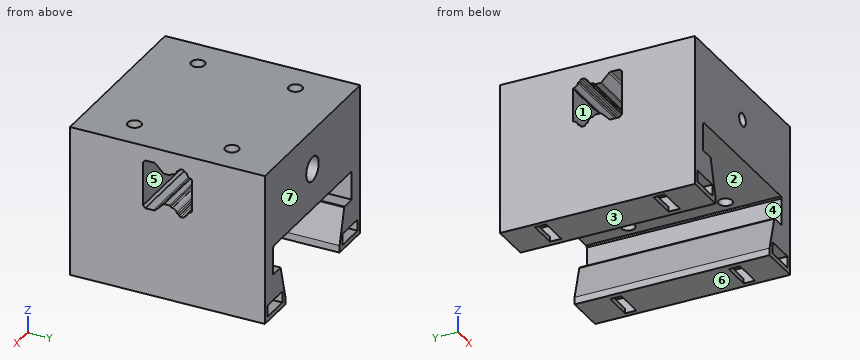
from build123d import *

# Parameters (mm, degrees)
SKETCH1_W           = 57
SKETCH1_H           = 28.7
BOSS_EXTRUDE1_DEPTH = 60
SKETCH2_W           = 9
SKETCH2_H           = 4
CUT_EXTRUDE1_DEPTH  = 69.064473112
BOSS_EXTRUDE2_DEPTH = 28.5
SKETCH6_W           = 15.5
SKETCH6_H           = 15.390476131
CUT_EXTRUDE2_DEPTH  = 80
BOSS_EXTRUDE5_DEPTH = 60
SKETCH10_R          = 2.1
CUT_EXTRUDE3_DEPTH  = 24.530533394
SKETCH11_W          = 61.984050455
SKETCH11_H          = 43.227353824
SKETCH11_W_2        = 6
SKETCH11_H_2        = 2.542732203
CUT_EXTRUDE4_DEPTH  = 77.839254789
SKETCH13_W          = 6.011053281
SKETCH13_H          = 2.620549071
CUT_EXTRUDE5_DEPTH  = 77.839254789
SKETCH14_W          = 9
SKETCH14_H          = 4
BOSS_EXTRUDE7_DEPTH = 60
SKETCH12_W          = 10.230058637
SKETCH12_H          = 6.686923691
BOSS_EXTRUDE6_DEPTH = 60
SKETCH15_W          = 9
SKETCH15_H          = 4
BOSS_EXTRUDE8_DEPTH = 60
SKETCH16_W          = 9
SKETCH16_H          = 1.78
CUT_EXTRUDE6_DEPTH  = 77.839254789
SKETCH17_W          = 25.75
SKETCH17_H          = 20.1006285
CUT_EXTRUDE7_DEPTH  = 77.839254789
SKETCH18_W          = 32.4
SKETCH18_H          = 12.613288226
CUT_EXTRUDE8_DEPTH  = 75.79485996
SKETCH19_W          = 57
SKETCH19_H          = 3.949842852
CUT_EXTRUDE9_DEPTH  = 75.79485996
SKETCH20_W          = 9
SKETCH20_H          = 3.5
CUT_EXTRUDE10_DEPTH = 75.79485996
SKETCH21_W          = 9
SKETCH21_H          = 3.5
CUT_EXTRUDE11_DEPTH = 1.5
SKETCH23_R          = 3.75
CUT_EXTRUDE12_DEPTH = 59.313986952
SKETCH24_R          = 2
CUT_EXTRUDE13_DEPTH = 59.313986952


with BuildPart() as part:
    # Sketch1 → Boss-Extrude1 (new body)
    with BuildSketch(Plane(origin=(0, 0, 0), x_dir=(1, 0, 0), z_dir=(0, 1, 0))):
        with Locations((0, -0.5)):
            Rectangle(SKETCH1_W, SKETCH1_H)
        Polygon((23.07, -9.85), (-23.07, -9.85), (-23.5, -9.42), (-23.5, -0.95), (-19.09385128, -0.95), (-19, -0.599742255), (-16.2, 9.85), (16.2, 9.85), (19, -0.599742255), (19.09385128, -0.95), (23.5, -0.95), (23.5, -2.9), (23.5, -9.42), align=None, mode=Mode.SUBTRACT)
    extrude(amount=BOSS_EXTRUDE1_DEPTH)

    # Sketch2 → Cut-Extrude1 (cut, through all)
    with BuildSketch(Plane.XZ):
        with Locations((24, -10.0706285)):
            Rectangle(SKETCH2_W, SKETCH2_H)
        with Locations((-24, -10.0706285)):
            Rectangle(SKETCH2_W, SKETCH2_H)
    extrude(amount=-CUT_EXTRUDE1_DEPTH, mode=Mode.SUBTRACT)

    # Sketch5 → Boss-Extrude2 (add, symmetric)
    with BuildSketch(Plane(origin=(0, 0, 0), x_dir=(0, 0, -1), z_dir=(1, 0, 0))):
        with BuildLine():
            Line((-14.85, 0), (-14.85, 23.200000017))
            Line((-14.85, 23.200000017), (-15.549999973, 22.50000003))
            Line((-15.549999973, 22.50000003), (-29.149999973, 22.50000003))
            Line((-29.149999973, 22.50000003), (-29.849999973, 23.20000003))
            Line((-29.849999973, 23.20000003), (-29.849999973, 25.743360053))
            ThreePointArc((-29.849999973, 25.743360053), (-29.773879502, 26.126043492), (-29.557106746, 26.450466847))
            Line((-29.557106746, 26.450466847), (-27.237157266, 28.770416328))
            ThreePointArc((-27.237157266, 28.770416328), (-27.150448162, 28.900185674), (-27.119999973, 29.053259055))
            Line((-27.119999973, 29.053259055), (-27.119999973, 30.615319642))
            ThreePointArc((-27.119999973, 30.615319642), (-27.150448164, 30.768393021), (-27.237157268, 30.898162365))
            Line((-27.237157268, 30.898162365), (-27.431588163, 31.09259326))
            ThreePointArc((-27.431588163, 31.09259326), (-27.613507965, 31.297692563), (-27.620638933, 31.57175403))
            ThreePointArc((-27.620638933, 31.57175403), (-28.017573243, 32.42857618), (-28.828543655, 32.91234062))
            ThreePointArc((-28.828543655, 32.91234062), (-29.01918836, 33.020436377), (-29.124259054, 33.212764861))
            Line((-29.124259054, 33.212764861), (-29.156235284, 33.354092333))
            ThreePointArc((-29.156235284, 33.354092333), (-29.24659278, 33.53064407), (-29.410649592, 33.642090719))
            Line((-29.410649592, 33.642090719), (-29.585724304, 33.70524196))
            ThreePointArc((-29.585724304, 33.70524196), (-29.777329878, 33.851609246), (-29.849999973, 34.081511694))
            Line((-29.849999973, 34.081511694), (-29.849999973, 34.837490602))
            ThreePointArc((-29.849999973, 34.837490602), (-29.772088513, 35.074680338), (-29.568705112, 35.219471078))
            Line((-29.568705112, 35.219471078), (-29.427668799, 35.263299846))
            ThreePointArc((-29.427668799, 35.263299846), (-29.25116358, 35.375371369), (-29.155313737, 35.561185593))
            Line((-29.155313737, 35.561185593), (-29.125010632, 35.702102112))
            ThreePointArc((-29.125010632, 35.702102112), (-29.020526118, 35.897067182), (-28.828406063, 36.006695082))
            ThreePointArc((-28.828406063, 36.006695082), (-28.025619489, 36.481556021), (-27.62403672, 37.32339358))
            ThreePointArc((-27.62403672, 37.32339358), (-27.540484938, 37.407225271), (-27.43605838, 37.46293655))
            Line((-27.43605838, 37.46293655), (-27.39899493, 37.5))
            Line((-27.39899493, 37.5), (-17.30100503, 37.5))
            Line((-17.30100503, 37.5), (-17.26394158, 37.46293655))
            ThreePointArc((-17.26394158, 37.46293655), (-17.159515017, 37.407225278), (-17.07596324, 37.32339358))
            ThreePointArc((-17.07596324, 37.32339358), (-16.674380468, 36.481556018), (-15.871593887, 36.006695079))
            ThreePointArc((-15.871593887, 36.006695079), (-15.679473839, 35.897067189), (-15.574989331, 35.702102127))
            Line((-15.574989331, 35.702102127), (-15.544686222, 35.561185587))
            ThreePointArc((-15.544686222, 35.561185587), (-15.448836377, 35.375371364), (-15.272331158, 35.263299843))
            Line((-15.272331158, 35.263299843), (-15.131294869, 35.219471083))
            ThreePointArc((-15.131294869, 35.219471083), (-14.927911462, 35.074680333), (-14.85, 34.837490586))
            Line((-14.85, 34.837490586), (-14.85, 60))
            Line((-14.85, 60), (-34.380533394, 60))
            Line((-34.380533394, 60), (-34.380533394, 0))
            Line((-34.380533394, 0), (-14.85, 0))
        make_face()
        with BuildLine():
            ThreePointArc((-15.142893227, 26.450466847), (-14.926120471, 26.126043492), (-14.85, 25.743360053))
            Line((-14.85, 25.743360053), (-14.85, 34.081511674))
            ThreePointArc((-14.85, 34.081511674), (-14.922670087, 33.851609245), (-15.114275644, 33.70524197))
            Line((-15.114275644, 33.70524197), (-15.289350386, 33.642090718))
            ThreePointArc((-15.289350386, 33.642090718), (-15.453407192, 33.53064407), (-15.543764688, 33.354092339))
            Line((-15.543764688, 33.354092339), (-15.57574092, 33.21276486))
            ThreePointArc((-15.57574092, 33.21276486), (-15.680811613, 33.020436377), (-15.871456319, 32.91234062))
            ThreePointArc((-15.871456319, 32.91234062), (-16.68242673, 32.42857618), (-17.07936104, 31.57175403))
            ThreePointArc((-17.07936104, 31.57175403), (-17.086492012, 31.297692565), (-17.26841181, 31.09259326))
            Line((-17.26841181, 31.09259326), (-17.462842708, 30.898162362))
            ThreePointArc((-17.462842708, 30.898162362), (-17.549551812, 30.768393016), (-17.58, 30.615319635))
            Line((-17.58, 30.615319635), (-17.58, 29.053259048))
            ThreePointArc((-17.58, 29.053259048), (-17.54955181, 28.900185669), (-17.462842705, 28.770416325))
            Line((-17.462842705, 28.770416325), (-15.142893227, 26.450466847))
        make_face()
    extrude(amount=BOSS_EXTRUDE2_DEPTH, both=True)

    # Sketch6 → Cut-Extrude2 (cut)
    with BuildSketch(Plane(origin=(0, 60, 0), x_dir=(1, 0, 0), z_dir=(0, 1, 0))):
        with Locations((0, 12.050145064)):
            Rectangle(SKETCH6_W, SKETCH6_H)
    extrude(amount=-CUT_EXTRUDE2_DEPTH, mode=Mode.SUBTRACT)

    # Sketch9 → Boss-Extrude5 (add)
    with BuildSketch(Plane(origin=(0, 60, 0), x_dir=(1, 0, 0), z_dir=(0, 1, 0))):
        Polygon((-19.5, 13.85), (-19.5, 29.1706285), (-28.5, 29.1706285), (-28.5, 26.1706285), (-33.5, 26.1706285), (-33.5, 32.1706285), (-14.5, 32.1706285), (-14.5, 13.85), align=None)
        Polygon((30.2, 12.85), (30.2, 28.735786438), (19.5, 28.735786438), (19.5, 13.85), (14.5, 13.85), (14.5, 32.1706285), (33.5, 32.1706285), (33.5, 12.85), align=None)
    extrude(amount=-BOSS_EXTRUDE5_DEPTH)

    # Sketch10 → Cut-Extrude3 (cut)
    with BuildSketch(Plane.XY.offset(34.380533394)):
        with Locations((19, 45)):
            Circle(SKETCH10_R)
        with Locations((19, 15)):
            Circle(SKETCH10_R)
        with Locations((-19, 15)):
            Circle(SKETCH10_R)
        with Locations((-19, 45)):
            Circle(SKETCH10_R)
    extrude(amount=-CUT_EXTRUDE3_DEPTH, mode=Mode.SUBTRACT)

    # Sketch11 → Cut-Extrude4 (cut, through all)
    with BuildSketch(Plane.XZ):
        with Locations((44.734239641, -35.463676912)):
            Rectangle(SKETCH11_W, SKETCH11_H)
        with Locations((32.2, -12.566438328)):
            Rectangle(SKETCH11_W_2, SKETCH11_H_2)
    extrude(amount=-CUT_EXTRUDE4_DEPTH, mode=Mode.SUBTRACT)


with BuildPart() as cut_extrude4_piece_1:
    # of the separate pieces the step leaves, piece 1, a body of its own (cut_extrude4_pieces)
    add(part.part.solids().sort_by_distance((-28.5, 23.200000017, 14.85))[0])

    # Sketch14 → Boss-Extrude7 (add, through all)
    with BuildSketch(Plane(origin=(0, 0, 0), x_dir=(-1, 0, 0), z_dir=(0, -1, 0))):
        with Locations((-24, 10.0706285)):
            Rectangle(SKETCH14_W, SKETCH14_H)
    extrude(amount=-BOSS_EXTRUDE7_DEPTH)

    # Sketch12 → Boss-Extrude6 (add, through all)
    with BuildSketch(Plane.XZ):
        with Locations((23.384970682, -10.506538155)):
            Rectangle(SKETCH12_W, SKETCH12_H)
    extrude(amount=-BOSS_EXTRUDE6_DEPTH)

    # Sketch15 → Boss-Extrude8 (add, through all)
    with BuildSketch(Plane(origin=(0, 60, 0), x_dir=(1, 0, 0), z_dir=(0, 1, 0))):
        with Locations((-24, 10.0706285)):
            Rectangle(SKETCH15_W, SKETCH15_H)
    extrude(amount=-BOSS_EXTRUDE8_DEPTH)

    # Sketch16 → Cut-Extrude6 (cut, through all)
    with BuildSketch(Plane(origin=(0, 60, 0), x_dir=(1, 0, 0), z_dir=(0, 1, 0))):
        with Locations((-24, 12.96)):
            Rectangle(SKETCH16_W, SKETCH16_H)
    extrude(amount=-CUT_EXTRUDE6_DEPTH, mode=Mode.SUBTRACT)

    # Sketch17 → Cut-Extrude7 (cut, through all)
    with BuildSketch(Plane(origin=(0, 60, 0), x_dir=(1, 0, 0), z_dir=(0, 1, 0))):
        with Locations((-20.625, 22.12031425)):
            Rectangle(SKETCH17_W, SKETCH17_H)
    extrude(amount=-CUT_EXTRUDE7_DEPTH, mode=Mode.SUBTRACT)

    # Sketch18 → Cut-Extrude8 (cut, through all)
    with BuildSketch(Plane(origin=(0, 60, 0), x_dir=(1, 0, 0), z_dir=(0, 1, 0))):
        with Locations((0, 16.156644113)):
            Rectangle(SKETCH18_W, SKETCH18_H)
    extrude(amount=-CUT_EXTRUDE8_DEPTH, mode=Mode.SUBTRACT)

    # Sketch19 → Cut-Extrude9 (cut, through all)
    with BuildSketch(Plane(origin=(0, 60, 0), x_dir=(1, 0, 0), z_dir=(0, 1, 0))):
        with Locations((0, 14.044921426)):
            Rectangle(SKETCH19_W, SKETCH19_H)
    extrude(amount=-CUT_EXTRUDE9_DEPTH, mode=Mode.SUBTRACT)

    # Sketch20 → Cut-Extrude10 (cut, through all)
    with BuildSketch(Plane(origin=(0, 60, 0), x_dir=(1, 0, 0), z_dir=(0, 1, 0))):
        with Locations((-22.5, 8.82)):
            Rectangle(SKETCH20_W, SKETCH20_H)
        with Locations((22.5, 8.82)):
            Rectangle(SKETCH20_W, SKETCH20_H)
    extrude(amount=-CUT_EXTRUDE10_DEPTH, mode=Mode.SUBTRACT)

    # Sketch21 → Cut-Extrude11 (cut)
    with BuildSketch(Plane(origin=(0, 0, -12.07), x_dir=(-1, 0, 0), z_dir=(0, 0, -1))):
        with Locations((-22.5, 48.25)):
            Rectangle(SKETCH21_W, SKETCH21_H)
        with Locations((22.5, 48.25)):
            Rectangle(SKETCH21_W, SKETCH21_H)
        with Locations((22.5, 11.75)):
            Rectangle(SKETCH21_W, SKETCH21_H)
        with Locations((-22.5, 11.75)):
            Rectangle(SKETCH21_W, SKETCH21_H)
    extrude(amount=-CUT_EXTRUDE11_DEPTH, mode=Mode.SUBTRACT)

    # Sketch23 → Cut-Extrude12 (cut, through all)
    with BuildSketch(Plane(origin=(0, 22.50000003, 0), x_dir=(1, 0, 0), z_dir=(0, 1, 0))):
        with Locations(Location((0, -22.349999973, 0), (0, 0, 90))):
            Circle(SKETCH23_R)
    extrude(amount=CUT_EXTRUDE12_DEPTH, mode=Mode.SUBTRACT)

    # Sketch24 → Cut-Extrude13 (cut, through all)
    with BuildSketch(Plane(origin=(0, 22.50000003, 0), x_dir=(1, 0, 0), z_dir=(0, 1, 0))):
        with Locations(Location((0, -22.349999973, 0), (0, 0, 270))):
            Circle(SKETCH24_R)
    extrude(amount=-CUT_EXTRUDE13_DEPTH, mode=Mode.SUBTRACT)


with BuildPart() as cut_extrude4_piece_2:
    # of the separate pieces the step leaves, piece 2, a body of its own (cut_extrude4_pieces)
    add(part.part.solids().sort_by_distance((33.5, 0, -13.85))[0])

    # Sketch13 → Cut-Extrude5 (cut, through all)
    with BuildSketch(Plane.XZ):
        with Locations((32.65361778, -14.054923964)):
            Rectangle(SKETCH13_W, SKETCH13_H)
    extrude(amount=-CUT_EXTRUDE5_DEPTH, mode=Mode.SUBTRACT)


solid = cut_extrude4_piece_1.part
Part model, mm, in its own coordinate system. Face numbers are marked on the shaded views. A direction names the side the tool comes from. Round coordinates to 2 decimals unless told otherwise and drop trailing zeros. Order: outer loops, then holes, each group sorted by start corner. A loop starts at its lowest first (then second) coordinate and runs counter-clockwise, first axis right, second up. Notation, with made-up numbers: (-9.75, -3.75) -> (-2.75, -3.75) arc R7 cw to (-2.75, 4.25) -> close; hole circle Ø9 at (-36, -7.5). An arc over 180 degrees is marked (long way). Put each result on its own line as item: value.
Q1. Band-saw the part on C-C (y = 28). Give the cut face in (x, z), and give its area (3 significant figures).
From the geometry:
outline: (-28.5, -12.07) -> (-16.2, -12.07) -> (-16.2, -9.85) -> (-19.09, 0.95) -> (-23.5, 0.95) -> (-23.5, 9.42) -> (-23.07, 9.85) -> (23.07, 9.85) -> (23.5, 9.42) -> (23.5, 0.95) -> (19.09, 0.95) -> (16.2, -9.85) -> (16.2, -12.07) -> (28.5, -12.07) -> (28.5, 16.69) -> (-28.5, 16.69) -> close; (-28.5, 28.01) -> (28.5, 28.01) -> (28.5, 34.38) -> (-28.5, 34.38) -> close; hole (-27, -10.57) -> (-18, -10.57) -> (-18, -7.07) -> (-27, -7.07) -> close; hole (18, -10.57) -> (27, -10.57) -> (27, -7.07) -> (18, -7.07) -> close
area: 1,070 mm2
Q2. Tool access for the marked faces 1, 2 and 3: list every direction of +Z, -Z, +X, -X, +Y, -Y with a clear straight run to the whole face (end or side of a thin tool).
From the geometry:
face 1: +X, -X
face 2: +Y, -Y
face 3: -Z, +X, -X, +Y, -Y
Q3. Band-saw the part on B-B (y = 45). State how many separate pieces and enclosed holes the cut face has, and give its area (3 significant figures).
From the geometry:
separate pieces: 3
enclosed holes: 3
area: 1,460 mm2
Q4. Pull direction Z, two halves, no side cores. Call the marked faces 4, 5, 6 and 7: pulls with the +Z half, pulls with the -Z half, needs draft (parallel to the pull), parting line crosses it, or undercut.
From the geometry:
face 4: undercut
face 5: undercut
face 6: pulls with the -Z half
face 7: needs draft
Q5. Band-saw the part on A-A (z = 22.35). Give the cut face in (x, y), and give its area (3 significant figures).
From the geometry:
outline: (-28.5, 0) -> (-2, 0) -> (-2, 22.5) -> (-28.5, 22.5) -> close; (-28.5, 37.5) -> (-3.75, 37.5) -> (-3.75, 60) -> (-28.5, 60) -> close; (2, 0) -> (28.5, 0) -> (28.5, 22.5) -> (2, 22.5) -> close; (3.75, 37.5) -> (28.5, 37.5) -> (28.5, 60) -> (3.75, 60) -> close; hole circle Ø4.2 at (-19, 15); hole circle Ø4.2 at (-19, 45); hole circle Ø4.2 at (19, 15); hole circle Ø4.2 at (19, 45)
area: 2,250 mm2
Q6. Pin check, flat tip, straight feed: pin 1 Ø1 at (x, z) = (14, 15.5) entering from -Y. Stop position of the tip, or through.
From the geometry:
pin 1: stops at y = 0
Q7. Wall check: line 1 (Z direction, x = -24, y = 30.5); line 2 (Y direction, x = -19, z = 22.25); line 3 (Z direction, x = 20, y = 42.5). Give the ranges that are in metal, low to high. Write a range as [from, to].
From the geometry:
line 1: z = [-12.07, -10.57], [-7.07, 17.58], [27.12, 34.38]
line 2: y = [0, 12.9], [17.1, 22.5], [37.5, 42.9], [47.1, 60]
line 3: z = [-12.07, -10.57], [-7.07, 0.95], [9.85, 34.38]
